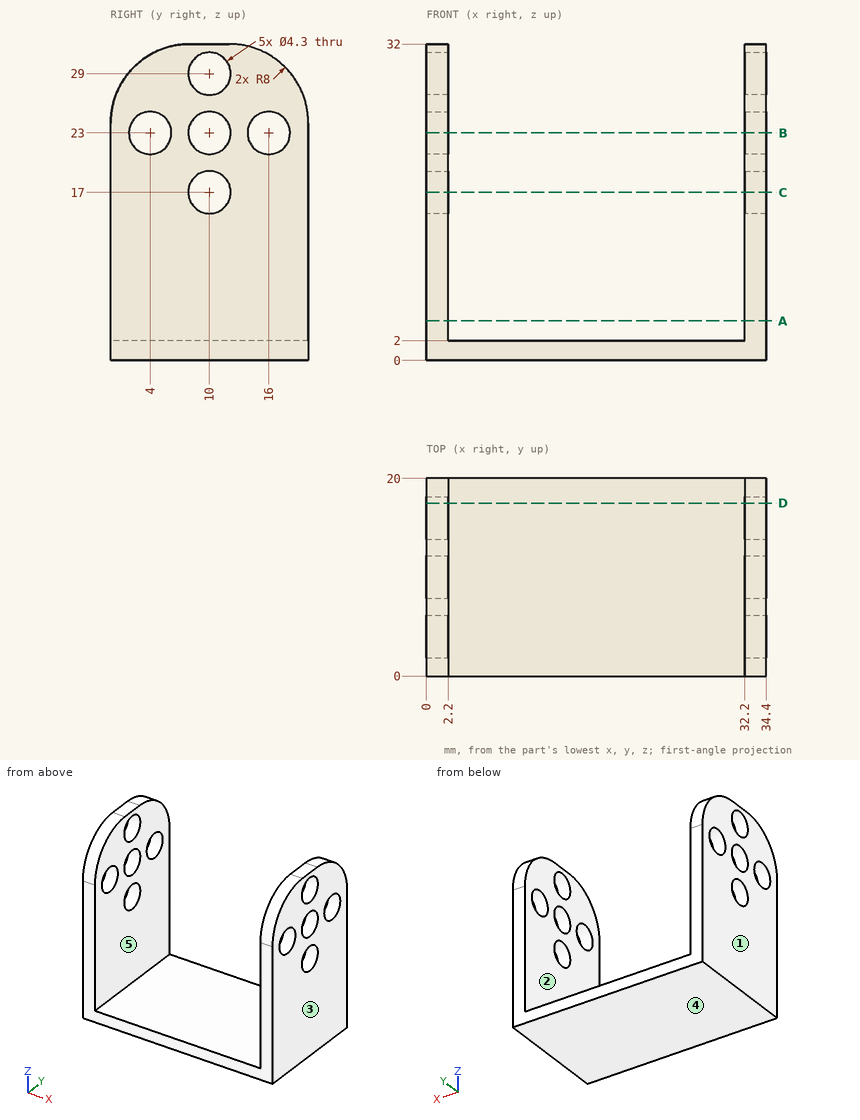
Verification items for this drawing (mm, ordinates from the low corner). A direction names the side the tool comes from. Coordinates: 2 decimals unless noted, no trailing zeros. Order: outer loops, then holes, each group sorted by start corner. A loop starts at its lowest first (then second) coordinate and runs counter-clockwise, first axis right, second up. Notation, with made-up numbers: (41.5, 79.25) - (76.5, 79.25) arc R17 cw to (76.5, 86.25) - close; hole circle Ø4 at (78.25, 71.5). An arc over 180 degrees is marked (long way). Answer as a JSON object with one key per item and string values. Group by question number.
Item 1: Sectioned sample at B-B, the plane z = 23. Give the number of separate pieces and of enclosed holes in the cut face, and give its area (3 significant figures).
Item 2: Scan lines: probe 1 along X at (y, z) = (10, 9); probe 2 along Y at (x, z) = (33, 17); probe 3 along Y at (x, z) = (32.8, 23). Record each from-to range of solid material in increasing order.
Item 3: Sectioned sample at C-C, the plane z = 17. Record the cut outline in (x, y), and give its area (3 significant figures).
Item 4: Sectioned sample at D-D, the plane y = 17.5. Record the cut outline in (x, z).
Item 5: Tool access check on the marked faces 4 and 5. Record the directions out of +Z, -Z, +X, -X, +Y, -Y that give a thin tool (end or side, any length) a straight path to the whole face; none if there is none.
Item 6: Draft check along X on the marked faces 1, 2 and 3. Enter one of: +X half, -X half, draft (parallel to the pull), parting line (faces both ways), or undercut.
Item 7: Sectioned sample at A-A, the plane z = 4. Record the cut outline in (x, y), and give its area (3 significant figures).
Resolved:
{
 "1": {"separate pieces": "8", "enclosed holes": "0", "area": "31.2 mm^2"},
 "2": {"probe 1": "0 to 2.2, 32.2 to 34.4", "probe 2": "0 to 7.85, 12.15 to 20", "probe 3": "0 to 1.85, 6.15 to 7.85, 12.15 to 13.85, 18.15 to 20"},
 "3": {"outline": "(0, 0) - (2.2, 0) - (2.2, 7.85) - (0, 7.85) - close; (0, 12.15) - (2.2, 12.15) - (2.2, 20) - (0, 20) - close; (32.2, 0) - (34.4, 0) - (34.4, 7.85) - (32.2, 7.85) - close; (32.2, 12.15) - (34.4, 12.15) - (34.4, 20) - (32.2, 20) - close", "area": "69.1 mm^2"},
 "4": {"outline": "(0, 0) - (34.4, 0) - (34.4, 21.46) - (32.2, 21.46) - (32.2, 2) - (2.2, 2) - (2.2, 21.46) - (0, 21.46) - close; (0, 24.54) - (2.2, 24.54) - (2.2, 29.81) - (0, 29.81) - close; (32.2, 24.54) - (34.4, 24.54) - (34.4, 29.81) - (32.2, 29.81) - close"},
 "5": {"face 4": "-Z, +X, -X, +Y, -Y", "face 5": "+Z, +Y, -Y"},
 "6": {"face 1": "-X half", "face 2": "undercut", "face 3": "+X half"},
 "7": {"outline": "(0, 0) - (2.2, 0) - (2.2, 20) - (0, 20) - close; (32.2, 0) - (34.4, 0) - (34.4, 20) - (32.2, 20) - close", "area": "88.0 mm^2"}
}
